```python
from build123d import *

# Parameters (mm, degrees)
ESQUISSE1_R         = 3.25
BOSS_EXTRU_1_DEPTH  = 2
BOSS_EXTRU_2_DEPTH  = 18
ESQUISSE3_R         = 4.5
ESQUISSE3_R_2       = 3.25
BOSS_EXTRU_3_DEPTH  = 8
ESQUISSE4_R         = 3.25
BOSS_EXTRU_4_DEPTH  = 1
BOSS_EXTRU_6_DEPTH  = 0.5
BOSS_EXTRU_7_DEPTH  = 0.5
BOSS_EXTRU_8_DEPTH  = 0.5
BOSS_EXTRU_9_DEPTH  = 0.5
ESQUISSE15_W        = 0.75
ESQUISSE15_H        = 4
ESQUISSE15_W_2      = 4
ESQUISSE15_H_2      = 0.75
BOSS_EXTRU_10_DEPTH = 6


with BuildPart() as part:
    # Esquisse1 → Boss.-Extru.1 (new body)
    with BuildSketch(Plane.XY):
        Polygon((0, 0), (-16, 0), (-16, 12), (-12, 16), (0, 16), align=None)
        with Locations((-8, 8)):
            Circle(ESQUISSE1_R, mode=Mode.SUBTRACT)
    extrude(amount=BOSS_EXTRU_1_DEPTH)

    # Esquisse2 → Boss.-Extru.2 (add)
    with BuildSketch(Plane.XY.offset(2)):
        Polygon((-16, 0), (0, 0), (0, 16), (-12, 16), (-16, 12), align=None)
        Polygon((-2, 2), (-2, 14), (-10.299397605, 14), (-14, 10.299397605), (-14, 2), align=None, mode=Mode.SUBTRACT)
    extrude(amount=BOSS_EXTRU_2_DEPTH)

    # Esquisse3 → Boss.-Extru.3 (add)
    with BuildSketch(Plane(origin=(0, 0, 0), x_dir=(-1, 0, 0), z_dir=(0, 0, -1))):
        with Locations((8, 8)):
            Circle(ESQUISSE3_R)
        with Locations((8, 8)):
            Circle(ESQUISSE3_R_2, mode=Mode.SUBTRACT)
    extrude(amount=BOSS_EXTRU_3_DEPTH)

    # Esquisse4 → Boss.-Extru.4 (add)
    with BuildSketch(Plane(origin=(0, 0, 0), x_dir=(-1, 0, 0), z_dir=(0, 0, -1))):
        Polygon((2.5, 5.328427125), (2.5, 10.671572875), (2.853553391, 10.318019485), (5.681980515, 13.146446609), (5.328427125, 13.5), (10.671572875, 13.5), (10.318019485, 13.146446609), (13.146446609, 10.318019485), (13.5, 10.671572875), (13.5, 5.328427125), (13.146446609, 5.681980515), (10.318019485, 2.853553391), (10.671572875, 2.5), (5.328427125, 2.5), (5.681980515, 2.853553391), (2.853553391, 5.681980515), align=None)
        with Locations((8, 8)):
            Circle(ESQUISSE4_R, mode=Mode.SUBTRACT)
    extrude(amount=BOSS_EXTRU_4_DEPTH)

    # Esquisse11 → Boss.-Extru.6 (add)
    with BuildSketch(Plane(origin=(-3.732233047, -3.732233047, 0), x_dir=(0, 0, 1), z_dir=(-0.707106781, -0.707106781, 0))):
        Polygon((0, 9.313708499), (-1, 9.313708499), (-2.326649916, 11.313708499), (-1, 13.313708499), (0, 13.313708499), align=None)
    extrude(amount=BOSS_EXTRU_6_DEPTH)

    # Esquisse12 → Boss.-Extru.7 (add)
    with BuildSketch(Plane(origin=(-4.267766953, 4.267766953, 0), x_dir=(0, 0, -1), z_dir=(0.707106781, -0.707106781, 0))):
        Polygon((0, 2), (1, 2), (2.326649916, 0), (1, -2), (0, -2), align=None)
    extrude(amount=BOSS_EXTRU_7_DEPTH)

    # Esquisse13 → Boss.-Extru.8 (add)
    with BuildSketch(Plane(origin=(3.732233047, 3.732233047, 0), x_dir=(0, 0, -1), z_dir=(0.707106781, 0.707106781, 0))):
        Polygon((0, 13.313708499), (1, 13.313708499), (2.326649916, 11.313708499), (1, 9.313708499), (0, 9.313708499), align=None)
    extrude(amount=BOSS_EXTRU_8_DEPTH)

    # Esquisse14 → Boss.-Extru.9 (add)
    with BuildSketch(Plane(origin=(-11.732233047, 11.732233047, 0), x_dir=(0, 0, 1), z_dir=(-0.707106781, 0.707106781, 0))):
        Polygon((0, -2), (-1, -2), (-2.326649916, 0), (-1, 2), (0, 2), align=None)
    extrude(amount=BOSS_EXTRU_9_DEPTH)

    # Esquisse15 → Boss.-Extru.10 (add)
    with BuildSketch(Plane.XY.offset(20)):
        with Locations((-14.375, 6.15)):
            Rectangle(ESQUISSE15_W, ESQUISSE15_H)
        with Locations((-8, 1.625)):
            Rectangle(ESQUISSE15_W_2, ESQUISSE15_H_2)
        with Locations((-1.625, 8)):
            Rectangle(ESQUISSE15_W, ESQUISSE15_H)
        with Locations((-6.15, 14.375)):
            Rectangle(ESQUISSE15_W_2, ESQUISSE15_H_2)
        Polygon((-10.437222619, 13.862174986), (-13.265649743, 11.033747861), (-13.795979829, 11.564077947), (-10.967552704, 14.392505072), align=None)
    extrude(amount=BOSS_EXTRU_10_DEPTH)


solid = part.part
```
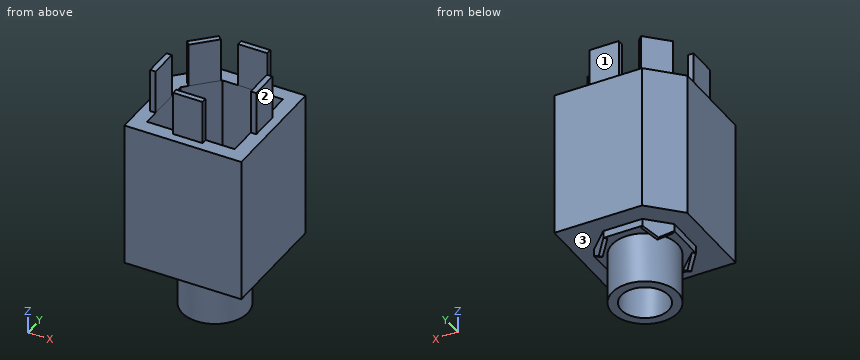
Build history of the part. All positions in model axes, mm. Face numbers are marked on the shaded views. A direction names the side the tool comes from. Round coordinates to 2 decimals unless told otherwise and drop trailing zeros. Loops run counter-clockwise (first coordinate to the right, second up) from the corner with the lowest first, then second, coordinate; pieces in that order, holes last.
Item 1: Pin check, flat tips, straight feed: P1, Ø0.5, axis at y = 9, z = -0.5, coming from the -X side; P2, Ø6, axis at x = -8.5, y = 6.5, coming from the +Z side; P3, Ø4.5, axis at x = -6, z = 22.5, coming from the -Y side; P4, Ø5, axis at x = -5.5, y = 7, coming from the -Z side. Stop position of each tip, or through.
Item 2: Saw through at A-A (z = 21). List the corners of the cut face in (x, y), then the cut area to 3 significant figures.
Item 3: Saw through at C-C (z = 13.5). List the corners of the cut face in (x, y).
Item 4: Saw through at D-D (z = -1.5). List the corners of the cut face in (x, y).
Item 5: Drill centre lines: line 1 along Y through (x, z) = (-8, -2.25); line 2 along X through (y, z) = (8, -0.3); line 3 along X through (y, z) = (8, 0.65). Where is each one in solid material? Low to high.
Item 6: Saw through at B-B (x = -7.25). List the corners of the cut face in (y, z).
Item 7: Which spindle directions (+Z, -Z, +X, -X, +Y, -Y) get a long thin tool onto all of the face, cutting with end or side? Do the marked faces 1, 2 and 3. Say none if no direction does.
Worked answers:
1. P1: stops at x = -13.5
1. P2: stops at z = 2
1. P3: stops at y = 1.25
1. P4: stops at z = -8
2. outline: (-14.75, 4.15) - (-14, 4.15) - (-14, 8.15) - (-14.75, 8.15) - close; (-13.8, 11.56) - (-13.27, 11.03) - (-10.44, 13.86) - (-10.97, 14.39) - close; (-10, 1.25) - (-6, 1.25) - (-6, 2) - (-10, 2) - close; (-8.15, 14) - (-4.15, 14) - (-4.15, 14.75) - (-8.15, 14.75) - close; (-2, 6) - (-1.25, 6) - (-1.25, 10) - (-2, 10) - close
2. area: 15.0 mm2
3. outline: (-16, 0) - (0, 0) - (0, 16) - (-12, 16) - (-16, 12) - close; hole (-14, 2) - (-2, 2) - (-2, 14) - (-10.3, 14) - (-14, 10.3) - close
4. outline: (-12.97, 4.8) - (-11.2, 3.03) - (-10.85, 3.39) - (-12.61, 5.15) - close; (-12.97, 11.2) - (-12.61, 10.85) - (-10.85, 12.61) - (-11.2, 12.97) - close; circle Ø9 at (-8, 8); (-5.15, 3.39) - (-4.8, 3.03) - (-3.03, 4.8) - (-3.39, 5.15) - close; (-5.15, 12.61) - (-3.39, 10.85) - (-3.03, 11.2) - (-4.8, 12.97) - close; hole circle Ø6.5 at (-8, 8)
5. line 1: y = 3.5 to 4.75, 11.25 to 12.5
5. line 2: x = -13.5 to -11.25, -4.75 to -2.5
5. line 3: x = -16 to -11.25, -4.75 to 0
6. outline: (0, 0) - (2.5, 0) - (2.5, -1) - (3.56, -1) - (3.56, -8) - (4.84, -8) - (4.84, 2) - (2, 2) - (2, 26) - (1.25, 26) - (1.25, 20) - (0, 20) - close; (11.16, -8) - (12.44, -8) - (12.44, -1) - (13.5, -1) - (13.5, 0) - (16, 0) - (16, 20) - (14.75, 20) - (14.75, 26) - (14, 26) - (14, 2) - (11.16, 2) - close
7. face 1: +Z, +X, -X, +Y
7. face 2: +Z, +X, +Y, -Y
7. face 3: -Z
